Design review of the part built by this model. Coordinates are the model's own, in mm. A direction names the side the tool comes from. Coordinates: 2 decimals unless noted, no trailing zeros. Write each loop counter-clockwise with the first axis right and the second up, starting at its lowest first coordinate (ties: lowest second). Pieces come first, ordered by that corner, then holes. Notation, with made-up numbers: M -28,-37.75 L 13,-37.75 A36 ccw 13,0.25 Z; hole C 80.25,5 d9. An arc over 180 degrees is marked long. One line per question, with ' | ' between items.
from build123d import *

# Parameters (mm, degrees)
SKETCH001_W        = 0.9
SKETCH001_H        = 0.3
POCKET_DEPTH       = 0.5
POLARPATTERN_COUNT = 12


with BuildPart() as part:
    # Sketch → Revolution (revolve)
    with BuildSketch(Plane.YZ):
        Polygon((-0.8, -6), (-2, -6), (-2, -1.1), (-4.5, -1.1), (-4.5, -0.1), (-2.6, -0.1), (-2.6, 0), (-1.1, 0), (-1.1, -3.5), (-0.8, -3.5), align=None)
    revolve(axis=Axis((0, 0, 0), (0, 0, 1)))

    # Sketch001 (on Face5 of Revolution) → Pocket (cut)
    with BuildSketch(Plane(origin=(0, 0, -0.1), x_dir=(0, -1, 0), z_dir=(0, 0, 1))):
        with Locations((0, 4.35)):
            Rectangle(SKETCH001_W, SKETCH001_H)
    pocket = extrude(amount=-POCKET_DEPTH, mode=Mode.SUBTRACT)

    # PolarPattern: Pocket ×12 about axis
    polarpattern_axis = Axis((0, 0, -0.1), (0, 0, 1))
    for i in range(1, POLARPATTERN_COUNT):
        add(pocket.rotate(polarpattern_axis, i * 360 / POLARPATTERN_COUNT), mode=Mode.SUBTRACT)


solid = part.part
1. Tool access review of faces 1 (the face through (-2, 1, -1.1)), 2 (the face through (2, 2, -0.1)), 3 (the face through (-1, -1, 0)): name each direction out of +Z, -Z, +X, -X, +Y, -Y from which nothing blocks a thin tool from reaching the whole face with its end or side.
Answer sheet:
face 1: -Z | face 2: +Z | face 3: +Z, +X, -X, +Y, -Y
2. Insertion check: pin 1 Ø0.7 at (x, y) = (0, 0) entering from +Z; pin 2 Ø1.5 at (y, z) = (-2, -1.5) entering from -X; pin 3 Ø2 at (x, y) = (0, 0) entering from +Z; pin 4 Ø1 at (x, z) = (0, -2.5) entering from +Y. Each pin has a flat end and moves straight along its axis. Give the tip position at first contact, or say it passes through.
Answer sheet:
pin 1: through | pin 2: x = -4.29 | pin 3: z = -3.5 | pin 4: y = 2
3. Draft analysis for pull direction Y (two halves, no side actions). For faces 4 (the face through (-0.49, 0.63, -4.77)), 5 (the face through (0, 1, -6)), 6 (the face through (1.352, -4.292, -0.593)), state which applies: pulls with the +Y half, pulls with the -Y half, needs draft (parallel to the pull), parting line crosses it, or undercut.
Answer sheet:
face 4: undercut | face 5: needs draft | face 6: parting line crosses it
4. Take a section at A-A (x = 0). Write out the cut boundary in (y, z), then the cut area to 3 significant figures.
Answer sheet:
outline: M -4.5,-1.1 L -2,-1.1 L -2,-6 L -0.8,-6 L -0.8,-3.5 L -1.1,-3.5 L -1.1,0 L -2.6,0 L -2.6,-0.1 L -4.2,-0.1 L -4.2,-0.6 L -4.5,-0.6 Z; M 0.8,-6 L 2,-6 L 2,-1.1 L 4.5,-1.1 L 4.5,-0.6 L 4.2,-0.6 L 4.2,-0.1 L 2.6,-0.1 L 2.6,0 L 1.1,0 L 1.1,-3.5 L 0.8,-3.5 Z | area: 17.1 mm^2
5. Take a section at D-D (y = -1.5). Write out the cut boundary in (x, z).
Answer sheet:
outline: M -4.24,-1.1 L -1.32,-1.1 L -1.32,-6 L 1.32,-6 L 1.32,-1.1 L 4.24,-1.1 L 4.24,-0.1 L 2.12,-0.1 L 2.12,0 L -2.12,0 L -2.12,-0.1 L -4.24,-0.1 Z
6. Take a section at C-C (z = -0.8). Write out the cut boundary in (x, y), then the cut area to 3 significant figures.
Answer sheet:
outline: C 0,0 d9; hole C 0,0 d2.2 | area: 59.8 mm^2
7. To check wall thickness, follow line 1 along X through (y, z) = (0, -0.75); line 2 along X through (y, z) = (0, -1.2); line 3 along Z through (x, y) = (-0.75, -3.25). State the ranges of each line that lie inside material, in increasing order. Write a range as [from, to].
Answer sheet:
line 1: [-4.5, -1.1], [1.1, 4.5] | line 2: [-2, -1.1], [1.1, 2] | line 3: [-1.1, -0.1]
